from build123d import *

# Parameters (mm, degrees)
SKETCH1_R           = 4.5
BOSS_EXTRUDE1_DEPTH = 8


with BuildPart() as part:
    # Sketch1 → Boss-Extrude1 (new body)
    with BuildSketch(Plane.XY):
        with BuildLine():
            Line((-119.390660592, 123.251708428), (-119.390660592, -10.748291572))
            ThreePointArc((-119.390660592, -10.748291572), (-117.047514842, -16.405145821), (-111.390660592, -18.748291572))
            Line((-111.390660592, -18.748291572), (-57.390660592, -18.748291572))
            ThreePointArc((-57.390660592, -18.748291572), (-51.733806343, -21.091437322), (-49.390660592, -26.748291572))
            Line((-49.390660592, -26.748291572), (-49.390660592, -40.748291572))
            Line((-49.390660592, -40.748291572), (-41.390660592, -48.748291572))
            Line((-41.390660592, -48.748291572), (149.609339408, -48.748291572))
            ThreePointArc((149.609339408, -48.748291572), (155.266193657, -46.405145821), (157.609339408, -40.748291572))
            Line((157.609339408, -40.748291572), (157.609339408, -23.201759464))
            ThreePointArc((157.609339408, -23.201759464), (156.599247983, -19.310592788), (153.824044881, -16.402034634))
            Line((153.824044881, -16.402034634), (-82.454216652, 130.051433259))
            ThreePointArc((-82.454216652, 130.051433259), (-84.477780716, 130.945790526), (-86.668922126, 131.251708428))
            Line((-86.668922126, 131.251708428), (-111.390660592, 131.251708428))
            ThreePointArc((-111.390660592, 131.251708428), (-117.047514842, 128.908562678), (-119.390660592, 123.251708428))
        make_face()
        with Locations((-99.390660592, 106.251708428)):
            Circle(SKETCH1_R, mode=Mode.SUBTRACT)
        with Locations((-99.390660592, 6.251708428)):
            Circle(SKETCH1_R, mode=Mode.SUBTRACT)
        with Locations((-17.390660592, -33.748291572)):
            Circle(SKETCH1_R, mode=Mode.SUBTRACT)
        with Locations((132.609339408, -33.748291572)):
            Circle(SKETCH1_R, mode=Mode.SUBTRACT)
    extrude(amount=BOSS_EXTRUDE1_DEPTH)


solid = part.part
The model under review builds one solid part; all positions refer to its coordinate system, in mm. A direction names the side the tool comes from. Coordinates: 2 decimals unless noted, no trailing zeros. Loops run counter-clockwise (first coordinate to the right, second up) from the corner with the lowest first, then second, coordinate; pieces in that order, holes last. Notation, with made-up numbers: M 23.5,-0.5 L 36.5,-0.5 A21 ccw 36.5,15.5 Z; hole C 21,74 d5. An arc over 180 degrees is marked long. Put each result on its own line as item: value. Start each with the question number.
Q1. Clearance check with flat-ended pins moving along their axes: pin 1 (8 mm diameter, centred on x = 3, y = 11.5, fed in from -Z); pin 2 (3 mm diameter, centred on y = 33, z = 4, fed in from +X). State where each tip first meets the part, or that it passes through.
Q2. The part is to be moulded in two halves that separate along Y. For faces 1 (the flat face through (-14, 23, 8)), 2 (the cylindrical face through (-14.971, -29.954, 3.944)), 3 (the flat face through (53, -48.748, 4)), 4 (the cylindrical face through (-95.098, 7.603, 3.944)), say which applies: +Y half, -Y half, draft (parallel to the pull), parting line (faces both ways), or undercut.
Q3. Add section B-B (x = 133). Write out the cut boundary in (y, z), and give its area (3 significant figures).
Q4. For faces 5 (the flat face through (-14, 23, 0)), 6 (the flat face through (-85, -18.748, 4)), list the 3-axis set-ups (+Z, -Z, +X, -X, +Y, -Y) from which the entire face can be reached by the end or side of a thin tool; tool diameter is ignored.
Q5. Add section D-D (x = -71.5). Write out the cut boundary in (y, z).
Q6. Add section C-C (y = -1). Write out the cut boundary in (x, z), and give its area (3 significant figures).
Q7. Wall thickness on line 1 (X direction, y = -37.5, z = 7); line 2 (X direction, y = 104, z = 6.25); line 3 (X direction, y = 69, z = 0.5): over which ranges is each line inside the solid? List them lowest first.
Q8. Add section A-A (z = 3.75). Write out the cut boundary in (x, y).
Answers:
1. pin 1: stops at z = 0
1. pin 2: stops at x = 76.54
2. face 1: draft
2. face 2: undercut
2. face 3: -Y half
2. face 4: undercut
3. outline: M -48.75,0 L -38.23,0 L -38.23,8 L -48.75,8 Z; M -29.27,0 L -3.49,0 L -3.49,8 L -29.27,8 Z
3. area: 290 mm^2
4. face 5: -Z, +X, -X, +Y, -Y
4. face 6: +Z, -Z, -X, -Y
5. outline: M -18.75,0 L 123.26,0 L 123.26,8 L -18.75,8 Z
6. outline: M -119.39,0 L 128.98,0 L 128.98,8 L -119.39,8 Z
6. area: 1,990 mm^2
7. line 1: x = -49.39 to -19.88, -14.91 to 130.12, 135.09 to 157.61
7. line 2: x = -119.39 to -103.29, -95.49 to -40.42
7. line 3: x = -119.39 to 16.04
8. outline: M -119.39,-10.75 A8 ccw -111.39,-18.75 L -57.39,-18.75 A8 cw -49.39,-26.75 L -49.39,-40.75 L -41.39,-48.75 L 149.61,-48.75 A8 ccw 157.61,-40.75 L 157.61,-23.2 A8 ccw 153.82,-16.4 L -82.45,130.05 A8 ccw -86.67,131.25 L -111.39,131.25 A8 ccw -119.39,123.25 Z; hole C -99.39,6.25 d9; hole C -99.39,106.25 d9; hole C -17.39,-33.75 d9; hole C 132.61,-33.75 d9
